from build123d import *

# Parameters (mm, degrees)
F0_R     = 22.7775322378
F1_DEPTH = 207.9115826637
F2_R     = 17.4342882966
F3_DEPTH = 52.1602202207
F4_SIZE2 = 50.8
F4_SIZE  = 7.62
F5_R     = 7.0950919486
F6_DEPTH = 295.2890638262


with BuildPart() as f1:
    # F0 (on Top) → F1 (new body)
    with BuildSketch(Plane.XY):
        with Locations((18.9419090748, 20.0417488813)):
            Circle(F0_R)
    extrude(amount=F1_DEPTH)

    # F2 (on face) → F3 (join)
    with BuildSketch(Plane.XY.offset(207.9115826637)):
        with Locations((18.9419090748, 20.0417488813)):
            Circle(F2_R)
    extrude(amount=F3_DEPTH)

    # F4
    f4_edges = [f1.edges().sort_by_distance(p)[0] for p in [
        (1.507621, 20.041749, 260.071803),
    ]]
    f4_side = f1.faces().sort_by_distance((18.941909, 20.041749, 260.071803))[0]
    chamfer(f4_edges, length=F4_SIZE, length2=F4_SIZE2, reference=f4_side)

    # F5 (on face) → F6 (cut)
    with BuildSketch(Plane.XY.offset(260.0718028843)):
        with Locations((18.9419090748, 20.0417488813)):
            Circle(F5_R)
    extrude(amount=-F6_DEPTH, mode=Mode.SUBTRACT)


solid = f1.part
Can you work these out from the model? Positions are in its coordinate system, mm. A direction names the side the tool comes from. Coordinates: 2 decimals unless noted, no trailing zeros. Write each loop counter-clockwise with the first axis right and the second up, starting at its lowest first coordinate (ties: lowest second). Pieces come first, ordered by that corner, then holes.
Q1. If we mould it in two halves opening along X, with no side actions, what happens to faces 1 (the face through (16, 27, 260.072)), 2 (the face through (29.452, -0.166, 102.5)), 3 (the face through (13.713, 24.837, 131.856))? For each: +X half, -X half, draft (parallel to the pull), parting line (faces both ways), or undercut.
Results found:
face 1: draft
face 2: parting line
face 3: undercut
Q2. For P1, Ø8, axis at x = 19, z = 221.5, coming from the -Y side; P2, Ø2, axis at x = 6, z = 173, coming from the -Y side; P3, Ø12, axis at x = 21.5, z = 186.5, coming from the -Y side, each with a flat end and sliding along its axis, tell me the tip position at first contact or that it passes through.
Results found:
P1: stops at y = 3.84
P2: stops at y = 0.65
P3: stops at y = -2.74
Q3. Please list where these lines run through material, in increasing order: L1, parallel to X at y = 22, z = 66.5; L2, parallel to X at y = 15.5, z = 209; L3, parallel to Z at x = 6.5, y = 3.
Results found:
L1: x = -3.75 to 12.12, 25.76 to 41.64
L2: x = 2.11 to 13.49, 24.39 to 35.77
L3: z = 0 to 207.91
Q4. Which directions (+Z, -Z, +X, -X, +Y, -Y) give clear straight access to the entire face, cutting with the end or side of a thin tool? Please do faces 4 (the face through (13.6, 25.4, 0)), 5 (the face through (35.57, 25.28, 208.58)).
Results found:
face 4: -Z, +X, -X, +Y, -Y
face 5: +Z
Q5. Imagine slicing it at A-A, the plane z = 177. List the corners of the cut face in (x, y) for me, plus the area to 3 significant figures.
Results found:
outline: circle Ø45.56 at (18.94, 20.04); hole circle Ø14.19 at (18.94, 20.04)
area: 1,470 mm2
Q6. Imagine slicing it at B-B, the plane x = 39. List the corners of the cut face in (y, z) for me.
Results found:
outline: (9.25, 0) - (30.83, 0) - (30.83, 207.91) - (9.25, 207.91) - close
